from build123d import *

# Parameters (mm, degrees)
F1_DEPTH      = 15
F2_R          = 1.5314851855
F3_DEPTH      = 12
F4_DEPTH      = 70
F4_DEPTH_BACK = 15
F5_START      = 15
F5_DEPTH      = 10


with BuildPart() as f1:
    # F0 (on Top) → F1 (new body)
    with BuildSketch(Plane.XY):
        with BuildLine():
            Line((-3.7878935624, 0), (0, 0))
            Line((0, 0), (10.080419369, 0))
            ThreePointArc((10.080419369, 0), (13.615953275, 1.4644660941), (15.080419369, 5))
            Line((15.080419369, 5), (15.080419369, 9.6347117797))
            Line((15.080419369, 9.6347117797), (0, 9.6347117797))
            Line((0, 9.6347117797), (2.9323033523, 19.0599747002))
            Line((2.9323033523, 19.0599747002), (30.7891890407, 19.0599747002))
            Line((30.7891890407, 19.0599747002), (30.7891890407, 24.113586992))
            ThreePointArc((30.7891890407, 24.113586992), (29.3247229466, 27.649120898), (25.7891890407, 29.113586992))
            Line((25.7891890407, 29.113586992), (-0.3710855943, 29.113586992))
            ThreePointArc((-0.3710855943, 29.113586992), (-3.1742094006, 28.2539368476), (-5.0134508929, 25.9705857625))
            Line((-5.0134508929, 25.9705857625), (-9.5392790792, 14.6563360963))
            ThreePointArc((-9.5392790792, 14.6563360963), (-4.3326845259, 14.6456991486), (-0.2697541602, 11.3897297337))
            Line((-0.2697541602, 11.3897297337), (-0.2609815599, 3.0549731831))
            ThreePointArc((-0.2609815599, 3.0549731831), (-1.7930786348, 1.2603868413), (-3.7878935624, 0))
        make_face()
    extrude(amount=F1_DEPTH)

    # F2 (on Right) → F3 (join)
    with BuildSketch(Plane.YZ):
        with Locations((13.9912003651, 4.9216861258)):
            Circle(F2_R)
    extrude(amount=F3_DEPTH)

    # F0 (on Top) → F4 (join, two sides)
    with BuildSketch(Plane.XY) as f4_sk:
        with BuildLine():
            Line((-6.2310085321, 0), (-3.7878935624, 0))
            ThreePointArc((-3.7878935624, 0), (-1.7930786348, 1.2603868413), (-0.2609815599, 3.0549731831))
            Line((-0.2609815599, 3.0549731831), (-0.2697541602, 11.3897297337))
            ThreePointArc((-0.2697541602, 11.3897297337), (-4.3326845259, 14.6456991486), (-9.5392790792, 14.6563360963))
            Line((-9.5392790792, 14.6563360963), (-10.8459586275, 11.3897298455))
            Line((-10.8459586275, 11.3897298455), (-10.845246293, 10.7129482743))
            ThreePointArc((-10.845246293, 10.7129482743), (-5.0783751094, 12.1030419278), (-1.7169344136, 7.215314433))
            ThreePointArc((-1.7169344136, 7.215314433), (-5.0732316586, 2.3295608244), (-10.8378749283, 3.7094910741))
            Line((-10.8378749283, 3.7094910741), (-10.8371860272, 3.0549732948))
            ThreePointArc((-10.8371860272, 3.0549732948), (-8.9945991742, 0.8331586588), (-6.2310085321, 0))
        make_face()
    extrude(amount=-F4_DEPTH)
    extrude(f4_sk.sketch, amount=F4_DEPTH_BACK)

    # F0 (on Top) → F5 (cut)
    with BuildSketch(Plane.XY.offset(F5_START)):
        with BuildLine():
            Line((-10.8392332305, 4.9999998882), (-10.8378749283, 3.7094910741))
            ThreePointArc((-10.8378749283, 3.7094910741), (-5.0732316586, 2.3295608244), (-1.7169344136, 7.215314433))
            ThreePointArc((-1.7169344136, 7.215314433), (-5.0783751094, 12.1030419278), (-10.845246293, 10.7129482743))
            Line((-10.845246293, 10.7129482743), (-10.8440068229, 9.5353405923))
            Line((-10.8440068229, 9.5353405923), (-7.9774604405, 9.5353405923))
            Line((-7.9774604405, 9.5353405923), (-7.9774604405, 4.9999998882))
            Line((-7.9774604405, 4.9999998882), (-10.8392332305, 4.9999998882))
        make_face()
        Polygon((-10.8440068229, 9.5353405923), (-10.8392332305, 4.9999998882), (-7.9774604405, 4.9999998882), (-7.9774604405, 9.5353405923), align=None)
    extrude(amount=F5_DEPTH, mode=Mode.SUBTRACT)


solid = f1.part
Source: CAD feature listing. Evaluate the final solid. Frame: model axes, mm. A direction names the side the tool comes from. Round coordinates to 2 decimals unless told otherwise and drop trailing zeros. Loops run counter-clockwise (first coordinate to the right, second up) from the corner with the lowest first, then second, coordinate; pieces in that order, holes last. Notation, with made-up numbers: (33.25, -10) -> (92.25, -10) arc R8 cw to (92.25, -2) -> close; hole circle Ø2 at (-19.5, -5). An arc over 180 degrees is marked (long way). Answer as a JSON object with one key per item and string values. Group by question number.
Q1. Section query D-D (x = 22.5). Output: boundary loops of the cut face in (y, z), plus the area to 3 significant figures.
Q2. Section query A-A (x = 8.5). Output: boundary loops of the cut face in (y, z).
Q3. Mould query, pull axis X, two halves, no side actions, for faces 5 (the cylindrical face through (-1.72, 7.4, -28.1)), 6 (the cylindrical face through (-9.029, 0.856, -28.095)), 7 (the flat face through (13, 29.114, 7)), 8 (the flat face through (30.789, 22, 7)). Classes: pulls with the +X half, pulls with the -X half, needs draft (parallel to the pull), parting line crosses it, or undercut.
Q4. Ray query, line 1 (Z direction, x = 14, y = 3.25); line 2 (X direction, y = 7.5, z = -4); line 3 (X direction, y = 12, z = -35). Return the intervals inside material, ascending. Write a range as from..to.
Q5. Section query C-C (y = 18.25). Output: boundary loops of the cut face in (x, z).
Q6. Contact query for flat-ended pins moving along their axis: P1, Ø14.5, axis at x = 18, y = 12, coming from the -Z side; P2, Ø1.5, axis at y = 14, z = 5, coming from the +X side; P3, Ø5, axis at y = 7.5, z = 9, coming from the +X side. Output: stop coordinate, or through.
Q7. Access query for faces 1 (the flat face through (12, 14, 5)), 2 (the cylindrical face through (-4.26, 14.62, -34.51)), 3 (the flat face through (15.08, 7, 7)), 4 (the cylindrical face through (-1.818, 1.239, -34.51)). Directions: +Z, -Z, +X, -X, +Y, -Y. A direction counts if a zero-diameter tool reaches every point of the face in a straight line with its end or side. Return the directions, or none.
Q8. Section query B-B (z = -36.5). Output: boundary loops of the cut face in (x, y), plus the area to 3 significant figures.
Completed:
{
 "1": {"outline": "(19.06, 0) -> (29.11, 0) -> (29.11, 15) -> (19.06, 15) -> close", "area": "151 mm²"},
 "2": {"outline": "(0, 0) -> (9.63, 0) -> (9.63, 15) -> (0, 15) -> close; circle Ø3.06 at (13.99, 4.92); (19.06, 0) -> (29.11, 0) -> (29.11, 15) -> (19.06, 15) -> close"},
 "3": {"face 5": "undercut", "face 6": "pulls with the -X half", "face 7": "needs draft", "face 8": "pulls with the +X half"},
 "4": {"line 1": "0..15", "line 2": "-1.72..-0.27", "line 3": "-10.6..-9.07, -4.83..-0.69"},
 "5": {"outline": "(-8.1, 0) -> (2.68, 0) -> (2.68, 15) -> (-8.1, 15) -> close"},
 "6": {"P1": "z = 0", "P2": "x = 12", "P3": "x = 15.08"},
 "7": {"face 1": "+Z, -Z, +X", "face 2": "-Z, +Y", "face 3": "+Z, -Z, +X, -Y", "face 4": "-Z, +X, -Y"},
 "8": {"outline": "(-10.85, 10.71) arc R5.23 cw (long way) to (-10.84, 3.71) -> (-10.84, 3.05) arc R5 ccw to (-6.23, 0) -> (-3.79, 0) arc R7.88 ccw to (-0.26, 3.05) -> (-0.27, 11.39) arc R7.88 ccw to (-9.54, 14.66) -> (-10.85, 11.39) -> close", "area": "61.5 mm²"}
}
